Autodesk Inventor part; units mm, degrees
ref_plane "YZ Plane" through (0, 0, 0) normal (1, 0, 0) x (0, 1, 0)
ref_plane "XZ Plane" through (0, 0, 0) normal (0, 1, 0) x (-1, 0, 0)
ref_plane "XY Plane" through (0, 0, 0) normal (0, 0, 1) x (1, 0, 0)
sketch "Boceto1" plane through (0, 0, 0) normal (0, 1, 0) x (-1, 0, 0)
  line L0 (-8, -15.55) -> (8, -15.55)
  line L1 (8, -15.55) -> (8, 15.55)
  line L2 (8, 15.55) -> (-8, 15.55)
  line L3 (-8, 15.55) -> (-8, -15.55)
  line L4 (-8, -15.55) -> (8, 15.55) construction
  line L5 (8, -15.55) -> (-8, 15.55) construction
  line L6 (9.5, 17.05) -> (9.5, -17.05)
  line L7 (9.5, -17.05) -> (-9.5, -17.05)
  line L8 (-9.5, -17.05) -> (-9.5, 17.05)
  line L9 (-9.5, 17.05) -> (9.5, 17.05)
  point P0 (0, 0)
  dimension "d0" = 16
  dimension "d1" = 31.1
  dimension "d2" = 1.5
extrude "Extrusión1" add sketch "Boceto1" along normal blind 6
sketch "Boceto2" plane through (0, 0, 0) normal (0, -1, 0) x (1, 0, 0)
  line L0 (9.5, 17.05) -> (9.5, -17.05)
  line L1 (-9.5, 17.05) -> (9.5, 17.05)
  line L2 (-9.5, -17.05) -> (-9.5, 17.05)
  line L3 (9.5, -17.05) -> (-9.5, -17.05)
  line L4 (8, -15.55) -> (8, 15.55)
  line L5 (-8, -15.55) -> (8, -15.55)
  line L6 (-8, 15.55) -> (-8, -15.55)
  line L7 (8, 15.55) -> (-8, 15.55)
  line L8 (10.5, 18.05) -> (10.5, -18.05)
  line L9 (10.5, -18.05) -> (-10.5, -18.05)
  line L10 (-10.5, -18.05) -> (-10.5, 18.05)
  line L11 (-10.5, 18.05) -> (10.5, 18.05)
  line L12 (10.5, -18.05) -> (-10.5, -18.05)
  line L13 (-10.5, -18.05) -> (-10.5, -24.55)
  line L14 (-10.5, -24.55) -> (10.5, -24.55)
  line L15 (10.5, -24.55) -> (10.5, -18.05)
  point P0 (0, 0)
  dimension "d5" = 2.5
  dimension "d19" = 6.5
extrude "Extrusión2" add sketch "Boceto2" against normal blind 1 contours L0 L3 L2 L1 | L8 L9 L10 L11
sketch "Boceto8" plane through (0, 0, 0) normal (0, -1, 0) x (1, 0, 0)
  line L0 (10.5, 18.05) -> (10.5, -18.05)
  line L1 (10.5, -18.05) -> (-10.5, -18.05)
  line L2 (-10.5, -18.05) -> (-10.5, -23.55)
  line L3 (-10.5, -23.55) -> (10.5, -23.55)
  line L4 (10.5, -23.55) -> (10.5, -18.05)
  point P0 (0, 0)
  dimension "d20" = 21
  dimension "d21" = 5.5
extrude "Extrusión7" add sketch "Boceto8" against normal blind 1
sketch "Boceto9" plane through (0, 6, 0) normal (0, 1, 0) x (1, 0, 0)
  line L0 (9.5, -17.05) -> (9.5, 17.05)
  line L1 (9.5, 17.05) -> (-9.5, 17.05)
  line L2 (-9.5, 17.05) -> (-9.5, -17.05)
  line L3 (-9.5, -17.05) -> (9.5, -17.05)
  line L4 (8, 15.55) -> (8, -15.55)
  line L5 (8, -15.55) -> (-8, -15.55)
  line L6 (-8, -15.55) -> (-8, 15.55)
  line L7 (-8, 15.55) -> (8, 15.55)
  line L8 (-10.5, -18.05) -> (10.5, -18.05)
  line L9 (10.5, -18.05) -> (10.5, 23.55)
  line L10 (-9.5, -17.05) -> (9.5, -17.05)
  line L11 (-9.5, 17.05) -> (-9.5, -17.05)
  line L12 (9.5, 17.05) -> (-9.5, 17.05)
  line L13 (9.5, -17.05) -> (9.5, 17.05)
  line L14 (-8, 15.55) -> (8, 15.55)
  line L15 (8, 15.55) -> (8, 21.35)
  line L16 (8, 21.35) -> (-8, 21.35)
  line L17 (-8, 21.35) -> (-8, 15.55)
  line L18 (-10.5, 23.55) -> (-10.5, -18.05)
  line L19 (10.5, 23.55) -> (-10.5, 23.55)
  point P0 (0, 0)
  point P1 (8, 15.55)
  dimension "d24" = 5.8
extrude "Extrusión8" cut sketch "Boceto9" against normal blind 5 contours L15 L7 L17 L1 | L1 L17 L16 L15
fillet "Empalme3" radius 2 4 edges at (-10.5, 0.5, 18.05) (10.5, 0.5, 18.05) (-10.5, 0.5, -23.55) (10.5, 0.5, -23.55)
fillet "Empalme4" radius 2 4 edges at (-9.5, 3.5, -17.05) (-9.5, 3.5, 17.05) (9.5, 3.5, 17.05) (9.5, 3.5, -17.05)
sketch "Boceto10" plane through (0, 0, 0) normal (0, -1, 0) x (1, 0, 0)
  line L0 (8, -15.55) -> (8, 15.55)
  line L1 (-8, -15.55) -> (8, -15.55)
  line L2 (8, 15.55) -> (5.6, 15.55)
  line L3 (5.6, 15.55) -> (5.6, -15.55)
  line L4 (5.6, -15.55) -> (8, -15.55)
  line L5 (8, -15.55) -> (8, 15.55)
  line L6 (-8, -15.55) -> (-5.6, -15.55)
  line L7 (-5.6, -15.55) -> (-5.6, 15.55)
  line L8 (-5.6, 15.55) -> (-8, 15.55)
  line L9 (-8, 15.55) -> (-8, -15.55)
  point P0 (0, 0)
  dimension "d29" = 2.4
  dimension "d30" = 2.4
  dimension "d31" = 31.1
extrude "Extrusión9" add sketch "Boceto10" against normal blind 0.5
properties part number "Pieza USB Tester"
Work out the finished part from the listing and answer in its coordinate system (mm). A direction names the side the tool comes from. Give positions to 0.01 mm unless a question says otherwise; leave off trailing zeros. Loops run counter-clockwise (first coordinate to the right, second up) from the corner with the lowest first, then second, coordinate; pieces in that order, holes last. Notation, with made-up numbers: (23, 21.5) -> (52, 21.5) arc R20 ccw to (52, 60.5) -> close; hole circle Ø1 at (59, -9). An arc over 180 degrees is marked (long way). Use a Markdown table: item, result. Add a question column.
1) The part is cut by section C-C, the plane y = 2.3. Determine the outline of the cut face in (x, z).
2) The part is cut by section D-D, the plane x = 6. Determine the outline of the cut face in (y, z).
3) Which of the six approach directions +Z, -Z, +X, -X, +Y, -Y give full straight-line access (tool end or side, diameter ignored) to faces 4 (the cylindrical face through (-9.092, 3.465, -16.324)), 5 (the cylindrical face through (9.07, 3.46, -16.35)), 6 (the cylindrical face through (-8.9, 3.46, 16.48)), 7 (the flat face through (9.5, 3, 0))?
4) Consider line 1 along X through (y, z) = (1.05, 9.5); line 2 along Z through (x, y) = (-0.5, 0.5); line 3 along X through (y, z) = (0.8, 6). Determine where each line is inside the solid, lowest interval first.
5) Each of these flat-tipped pins is pushed along its axis until it touches: P1, Ø8, axis at x = 1.5, z = -4, coming from the +Y side; P2, Ø2, axis at y = 2.5, z = 2, coming from the -X side; P3, Ø3, axis at y = 3.5, z = -8, coming from the +X side; P4, Ø0.7, axis at x = 6.5, z = 7.5, coming from the +Y side. Where does it stop, or does it pass through?
6) For a pull along Z with two mould halves and no side action, classify faces 1 (the flat face through (-7, 0.5, 0)), 2 (the cylindrical face through (-9.93, 0.51, 17.45)), 3 (the flat face through (-0.1, 0.5, -23.55)) as +Z half, -Z half, draft (parallel to the pull), parting line (faces both ways), or undercut.
7) The part is cut by section B-B, the plane x = -4.75. Determine the outline of the cut face in (y, z), plus the area to 3 significant figures.
8) The part is cut by section A-A, the plane z = -12. Determine the outline of the cut face in (x, y), plus the area to 3 significant figures.
Reported:
| question | item | result |
|---|---|---|
| 1 | outline | (-9.5, -15.11) arc R2 ccw to (-8, -17.05) -> (-8, 15.55) -> (8, 15.55) -> (8, -17.05) arc R2 ccw to (9.5, -15.11) -> (9.5, 15.05) arc R2 ccw to (7.5, 17.05) -> (-7.5, 17.05) arc R2 ccw to (-9.5, 15.05) -> close |
| 2 | outline | (0, -23.55) -> (1, -23.55) -> (1, -15.55) -> (0.5, -15.55) -> (0.5, 15.55) -> (6, 15.55) -> (6, 17.05) -> (1, 17.05) -> (1, 18.05) -> (0, 18.05) -> close |
| 3 | face 4 | -Z, -X, +Y |
| 3 | face 5 | -Z, +X, +Y |
| 3 | face 6 | +Z, -X, +Y |
| 3 | face 7 | +Z, -Z, +X, +Y |
| 4 | line 1 | x = -9.5 to -8, 8 to 9.5 |
| 4 | line 2 | z = -23.55 to -15.55, 15.55 to 18.05 |
| 4 | line 3 | x = -10.5 to -8, 8 to 10.5 |
| 5 | P1 | passes through |
| 5 | P2 | stops at x = -9.5 |
| 5 | P3 | stops at x = 9.5 |
| 5 | P4 | stops at y = 0.5 |
| 6 | face 1 | undercut |
| 6 | face 2 | +Z half |
| 6 | face 3 | -Z half |
| 7 | outline | (0, -23.55) -> (1, -23.55) -> (1, -15.55) -> (0, -15.55) -> close; (0, 15.55) -> (6, 15.55) -> (6, 17.05) -> (1, 17.05) -> (1, 18.05) -> (0, 18.05) -> close |
| 7 | area | 18.0 mm^2 |
| 8 | outline | (-10.5, 0) -> (-5.6, 0) -> (-5.6, 0.5) -> (-8, 0.5) -> (-8, 6) -> (-9.5, 6) -> (-9.5, 1) -> (-10.5, 1) -> close; (5.6, 0) -> (10.5, 0) -> (10.5, 1) -> (9.5, 1) -> (9.5, 6) -> (8, 6) -> (8, 0.5) -> (5.6, 0.5) -> close |
| 8 | area | 22.4 mm^2 |
